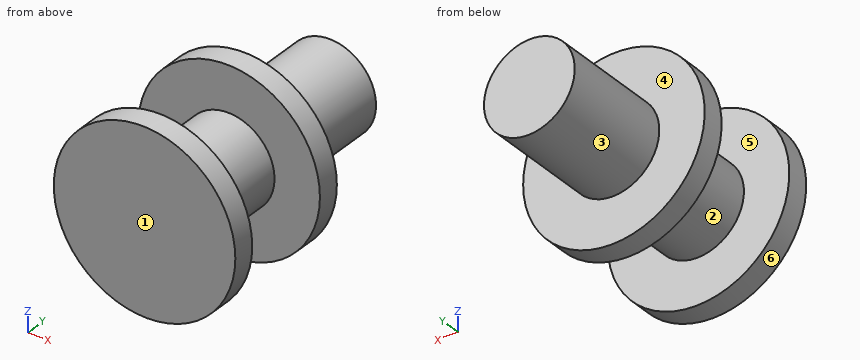
Autodesk Inventor part; units mm, degrees
ref_plane "Work Plane1" through (0, 0, 0) normal (0, 1, 0) x (1, 0, 0)
ref_plane "Work Plane6" through (-51.624, -18.8821, -44.9646) normal (1, 0, 0) x (0, 1, 0)
ref_plane "YZ Plane" through (0, 0, 0) normal (1, 0, 0) x (0, 1, 0)
ref_plane "Work Plane4" through (0, 152.4, 0) normal (0, 1, 0) x (1, 0, 0)
ref_plane "Work Plane5" through (0, 152.4, 0) normal (0, 1, 0) x (1, 0, 0)
ref_plane "Work Plane3" through (0, 152.4, 0) normal (0, -1, 0) x (1, 0, 0)
sketch "Sketch6" plane through (0, 152.4, 0) normal (0, -1, 0) x (1, 0, 0)
  circle A0 centre (0, 0) radius 104.5589
  circle A1 centre (0, 0) radius 50.8
  dimension "d15" = 101.6
extrude "Extrusion6" add sketch "Sketch6" along normal blind 254 contours A1
sketch "Sketch7" plane through (0, -101.6, 0) normal (0, -1, 0) x (1, 0, 0)
  circle A0 centre (0, 0) radius 104.5589
  circle A1 centre (0, 0) radius 101.6
  dimension "d18" = 203.2
extrude "Extrusion7" add sketch "Sketch7" along normal blind 25.4 contours A1
ref_plane "Work Plane1" through (0, 0, 0) normal (0, 1, 0) x (1, 0, 0)
sketch "Sketch8" plane through (0, 0, 0) normal (0, 1, 0) x (1, 0, 0)
  circle A0 centre (0, 0) radius 101.6
  dimension "d22" = 203.2
extrude "Extrusion8" add sketch "Sketch8" along normal blind 25.4
ref_plane "Work Plane2" through (75.376, -18.8821, -44.9646) normal (1, 0, 0) x (0, 1, 0)
sketch "Sketch9" plane through (75.376, -18.8821, -44.9646) normal (1, 0, 0) x (0, 1, 0)
  circle A0 centre (-604.603, 44.9646) radius 12.7
  point P0 (18.8821, 44.9646)
  dimension "d25" = 25.4
extrude "Extrusion9" cut sketch "Sketch9" against normal through all
ref_plane "Work Plane6" through (-51.624, -18.8821, -44.9646) normal (1, 0, 0) x (0, 1, 0)
properties part number "CapstanBottom-ver1-1111-2021"
For this review, take the finished solid that the model builds, in its own axes (mm). Face numbers are marked on the shaded views. A direction names the side the tool comes from. Round coordinates to 2 decimals unless told otherwise and drop trailing zeros. Write each loop counter-clockwise with the first axis right and the second up, starting at its lowest first coordinate (ties: lowest second). Pieces come first, ordered by that corner, then holes. Notation, with made-up numbers: (32.5, -11) - (67.5, -11) arc R22 ccw to (67.5, 23) - close; hole circle Ø4 at (28.25, 62). An arc over 180 degrees is marked (long way). Answer as CSV lines item,"result". Start each with the question number.
(1) Add section D-D, the plane y = 112.5. State the section outline as (x, z) points, plus the area to 3 significant figures.
(2) Add section B-B, the plane z = 0. State the section outline as (x, y) points.
(3) Add section A-A, the plane x = 0. State the section outline as (y, z) points.
(4) Machinability: for the marked faces 4, 5 and 6, which of the approach directions +Z, -Z, +X, -X, +Y, -Y give a long, thin tool a straight path to every point of the face, cutting with its end or side? Answer none if there is none.
(5) For line 1 (Y direction, x = -76.5, z = 1); line 2 (Z direction, x = 1.5, y = 138); line 3 (X direction, y = -9.5, z = -35), list the stretches that pass through material, from the lowest coordinate up.
(6) Mouldability with a two-part tool opening along Y and no side actions: class the marked faces 1, 2 and 3 as +Y half, -Y half, draft (parallel to the pull), parting line (faces both ways), or undercut.
(7) Add section C-C, the plane x = -66. State the section outline as (y, z) points.
(8) For pin 1 (5 mm diameter, centred on x = 10, y = 23, fed in from +Z); pin 2 (10 mm diameter, centred on x = -63.5, y = -1.5, fed in from +Z); pin 3 (12 mm diameter, centred on x = -57, y = 65, fed in from -Z); pin 4 (5 mm diameter, centred on x = -71.5, z = 73, fed in from +Y), all flat-tipped, find the tip position at first contact; note any pin that passes through.
From the geometry:
1,outline,"circle Ø101.6 at (0, 0)"
1,area,"8,110 mm²"
2,outline,"(-101.6, -127) - (101.6, -127) - (101.6, -101.6) - (50.8, -101.6) - (50.8, 0) - (101.6, 0) - (101.6, 25.4) - (50.8, 25.4) - (50.8, 152.4) - (-50.8, 152.4) - (-50.8, 25.4) - (-101.6, 25.4) - (-101.6, 0) - (-50.8, 0) - (-50.8, -101.6) - (-101.6, -101.6) - close"
3,outline,"(-127, -101.6) - (-101.6, -101.6) - (-101.6, -50.8) - (0, -50.8) - (0, -101.6) - (25.4, -101.6) - (25.4, -50.8) - (152.4, -50.8) - (152.4, 50.8) - (25.4, 50.8) - (25.4, 101.6) - (0, 101.6) - (0, 50.8) - (-101.6, 50.8) - (-101.6, 101.6) - (-127, 101.6) - close"
4,face 4,"+Y"
4,face 5,"none"
4,face 6,"+Y, -Y"
5,line 1,"y = -127 to -101.6, 0 to 25.4"
5,line 2,"z = -50.78 to 50.78"
5,line 3,"x = -36.82 to 36.82"
6,face 1,"-Y half"
6,face 2,"undercut"
6,face 3,"draft"
7,outline,"(-127, -77.24) - (-101.6, -77.24) - (-101.6, 77.24) - (-127, 77.24) - close; (0, -77.24) - (25.4, -77.24) - (25.4, 77.24) - (0, 77.24) - close"
8,pin 1,"stops at z = 101.32"
8,pin 2,"stops at z = 82.91"
8,pin 3,"passes through"
8,pin 4,"stops at y = 25.4"
